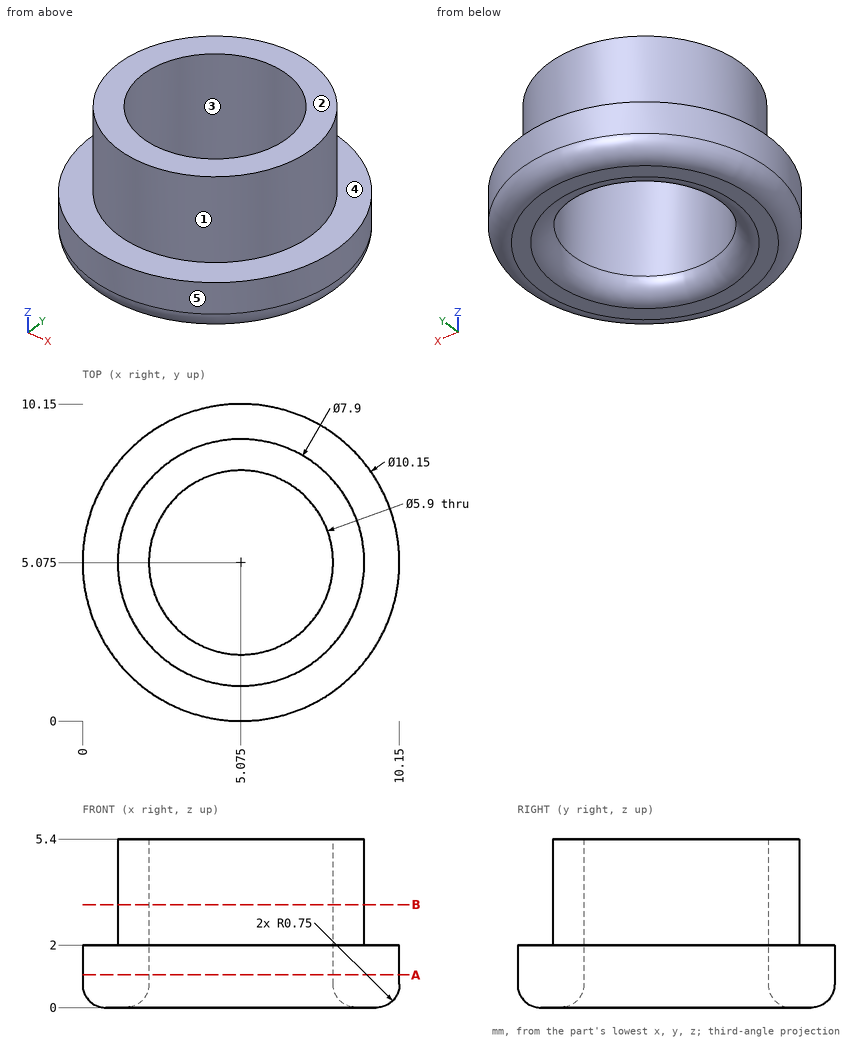
For this review, use the dimensioned drawing (mm, ordinates from the lowest corner) and the shaded views. A direction names the side the tool comes from. Round coordinates to 2 decimals unless told otherwise and drop trailing zeros. Order: outer loops, then holes, each group sorted by start corner. A loop starts at its lowest first (then second) coordinate and runs counter-clockwise, first axis right, second up. Notation, with made-up numbers: (39, 42) -> (63, 42) arc R13 cw to (63, 49) -> close; hole circle Ø5 at (20.25, 39.5). An arc over 180 degrees is marked (long way). One line per item, written item: value. Start each with the question number.
Q1. Take a section at A-A (z = 1.05). Write out the cut boundary in (x, y) (3 decimals), and give its area (3 significant figures).
Q2. Mouldability with a two-part tool opening along X and no side actions: class the marked faces 1, 2 and 3 as released by +X, released by -X, zero draft, split by the parting line, or undercut.
Q3. Machinability: for the marked faces 4 and 5, which of the approach directions +Z, -Z, +X, -X, +Y, -Y give a long, thin tool a straight path to every point of the face, cutting with its end or side? Answer none if there is none.
Q4. Wall thickness on line 1 (Y direction, x = 5, z = 1); line 2 (Z direction, x = 1, y = 5.5); line 3 (X direction, y = 7, z = 2.65): over which ranges is each line inside the solid? List them lowest first.
Q5. Clearance check with flat-ended pins moving along their axes: pin 1 Ø2 at (x, y) = (5, 5.5) entering from +Z; pin 2 Ø1 at (y, z) = (6.5, 1.5) entering from +X (3 decimals); pin 3 Ø1.5 at (x, z) = (9, 2) entering from -Y. State where each tip first meets the part, or that it passes through.
Q6. Take a section at B-B (z = 3.3). Write out the cut boundary in (x, y) (3 decimals), and give its area (3 significant figures).
Reported:
1. outline: circle Ø10.15 at (5.075, 5.075); hole circle Ø5.9 at (5.075, 5.075)
1. area: 53.6 mm2
2. face 1: split by the parting line
2. face 2: zero draft
2. face 3: undercut
3. face 4: +Z
3. face 5: +Z, -Z
4. line 1: y = 0 to 2.13, 8.02 to 10.15
4. line 2: z = 0 to 2
4. line 3: x = 1.63 to 2.84, 7.31 to 8.52
5. pin 1: passes through
5. pin 2: stops at x = 10.065
5. pin 3: stops at y = 1.12
6. outline: circle Ø7.9 at (5.075, 5.075); hole circle Ø5.9 at (5.075, 5.075)
6. area: 21.7 mm2
